```python
from build123d import *

# Parameters (mm, degrees)
SKETCH_R      = 4.75
PAD_DEPTH     = 1.9
SKETCH001_R   = 5.85
SKETCH001_R_2 = 4.75
PAD001_DEPTH  = 56
FILLET_R      = 4


with BuildPart() as part:
    # Sketch → Pad (new body)
    with BuildSketch(Plane.XY):
        with BuildLine():
            ThreePointArc((11, 4.75), (0, 6.523505), (-11, 4.75))
            ThreePointArc((-11, 4.75), (-11.771947, 0), (-11, -4.75))
            ThreePointArc((-11, -4.75), (0, -6.523505), (11, -4.75))
            ThreePointArc((11, -4.75), (11.771947, 0), (11, 4.75))
        make_face()
        Circle(SKETCH_R, mode=Mode.SUBTRACT)
    extrude(amount=PAD_DEPTH)

    # Sketch001 → Pad001 (join)
    with BuildSketch(Plane.XY):
        Circle(SKETCH001_R)
        Circle(SKETCH001_R_2, mode=Mode.SUBTRACT)
    extrude(amount=-PAD001_DEPTH)

    # Fillet
    fillet_edges = [part.edges().sort_by_distance(p)[0] for p in [
        (11, -4.75, 0.95),
        (-11, -4.75, 0.95),
        (-11, 4.75, 0.95),
        (11, 4.75, 0.95),
    ]]
    fillet(fillet_edges, radius=FILLET_R)


solid = part.part
```
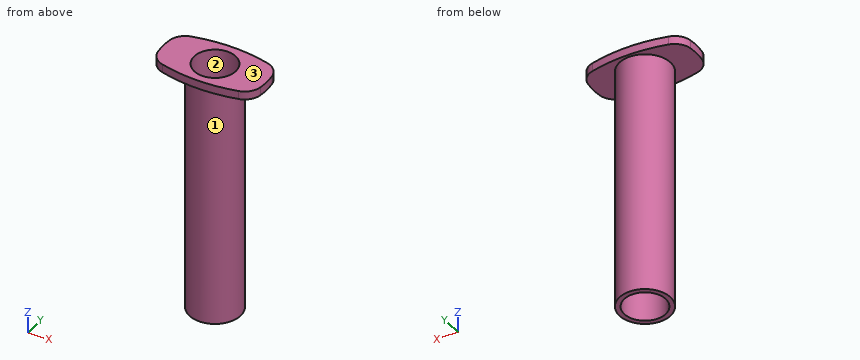
Geometry check sheet. Reference: the model listing, model coordinates, mm. Face numbers are marked on the shaded views. Give positions to 0.01 mm unless a question says otherwise; leave off trailing zeros. Write each loop counter-clockwise with the first axis right and the second up, starting at its lowest first coordinate (ties: lowest second). Pieces come first, ordered by that corner, then holes. Notation, with made-up numbers: (19, 26) -> (60, 26) arc R26 cw to (60, 44) -> close; hole circle Ø10 at (59, 44). An arc over 180 degrees is marked (long way). Use one line per item in the form item = value.
Item 1: Scan lines: line 1 (Y direction, x = 0, z = -42); line 2 (Z direction, x = -5.75, y = 3); line 3 (Y direction, x = 3.25, z = -17). Record each from-to range of solid material in increasing order.
Results list:
line_1 = -5.85 to -4.75, 4.75 to 5.85
line_2 = 0 to 1.9
line_3 = -4.86 to -3.46, 3.46 to 4.86
Item 2: Sectioned sample at D-D on x = -6.5. Enter the section's corners in (y, z).
Results list:
outline = (-5.91, 0) -> (5.91, 0) -> (5.91, 1.9) -> (-5.91, 1.9) -> close
Item 3: Sectioned sample at B-B on x = 0. Enter the section's corners in (y, z), plus the area to 3 significant figures.
Results list:
outline = (-6.52, 0) -> (-5.85, 0) -> (-5.85, -56) -> (-4.75, -56) -> (-4.75, 1.9) -> (-6.52, 1.9) -> close; (4.75, -56) -> (5.85, -56) -> (5.85, 0) -> (6.52, 0) -> (6.52, 1.9) -> (4.75, 1.9) -> close
area = 130 mm2
Item 4: Sectioned sample at C-C on z = -7. Enter the section's corners in (x, y).
Results list:
outline = circle Ø11.7 at (0, 0); hole circle Ø9.5 at (0, 0)
Item 5: Sectioned sample at A-A on y = 0. Enter the section's corners in (x, z), plus the area to 3 significant figures.
Results list:
outline = (-11.77, 0) -> (-5.85, 0) -> (-5.85, -56) -> (-4.75, -56) -> (-4.75, 1.9) -> (-11.77, 1.9) -> close; (4.75, -56) -> (5.85, -56) -> (5.85, 0) -> (11.77, 0) -> (11.77, 1.9) -> (4.75, 1.9) -> close
area = 150 mm2
Item 6: Depth check by flat-ended pin: pin 1 Ø3 at (y, z) = (2.5, -32) entering from -X; pin 2 Ø3 at (x, y) = (1.5, -2) entering from -Z (3 decimals); pin 3 Ø4 at (x, y) = (-1.5, -3) entering from -Z; pin 4 Ø8 at (x, z) = (-1, -29) entering from -Y. Enter the tip coordinate at first touch or a pass-through.
Results list:
pin_1 = -5.76
pin_2 = through
pin_3 = -56
pin_4 = -5.85
Item 7: Mould release check, pull along X, two halves, no side actions. Record for the marked faces 1, 2 and 3: released by +X, released by -X, zero draft, split by the parting line, or undercut.
Results list:
face_1 = split by the parting line
face_2 = undercut
face_3 = zero draft
